from build123d import *

# Parameters (mm, degrees)
F0_R     = 8.25
F1_DEPTH = 8


with BuildPart() as f1:
    # F0 (on Top) → F1 (new body)
    with BuildSketch(Plane.XY):
        with BuildLine():
            Line((-16, 18.282857), (-16, 12))
            ThreePointArc((-16, 12), (0, -20), (16, 12))
            Line((16, 12), (16, 18.282857))
            Line((16, 18.282857), (14, 18.282857))
            Line((14, 18.282857), (14, 14.282857))
            ThreePointArc((14, 14.282857), (10.5, 13.156254), (7, 14.282857))
            Line((7, 14.282857), (7, 18.282857))
            Line((7, 18.282857), (5, 18.282857))
            Line((5, 18.282857), (5, 14.282857))
            Line((5, 14.282857), (0, 14.282857))
            Line((0, 14.282857), (-5, 14.282857))
            Line((-5, 14.282857), (-5, 18.282857))
            Line((-5, 18.282857), (-7, 18.282857))
            Line((-7, 18.282857), (-7, 14.282857))
            ThreePointArc((-7, 14.282857), (-10.5, 13.156254), (-14, 14.282857))
            Line((-14, 14.282857), (-14, 18.282857))
            Line((-14, 18.282857), (-16, 18.282857))
        make_face()
        Circle(F0_R, mode=Mode.SUBTRACT)
    extrude(amount=F1_DEPTH)


solid = f1.part
Geometry: final body of the model. Coordinates: model frame, mm. A direction names the side the tool comes from. Round coordinates to 2 decimals unless told otherwise and drop trailing zeros. Order: outer loops, then holes, each group sorted by start corner. A loop starts at its lowest first (then second) coordinate and runs counter-clockwise, first axis right, second up.
Q1. Section D-D, the plane y = 0. Output: boundary loops of the cut face in (x, z), and give its area (3 significant figures).
Result sheet:
outline: (-20, 0) - (-8.25, 0) - (-8.25, 8) - (-20, 8) - close; (8.25, 0) - (20, 0) - (20, 8) - (8.25, 8) - close
area: 188 mm2
Q2. Pin query (flat end, axial travel): pin 1 (4 mm diameter, centred on x = 2.5, z = 2.5, fed in from +Y); pin 2 (4 mm diameter, centred on x = 5, z = 3, fed in from -Y); pin 3 (1.2 mm diameter, centred on y = 16, z = 2, fed in from +X); pin 4 (13 mm diameter, centred on x = 0, y = 0, fed in from -Z). Return the tip coordinate at first contact, or that it passes through.
Result sheet:
pin 1: stops at y = 14.28
pin 2: stops at y = -19.77
pin 3: stops at x = 16
pin 4: passes through
Q3. Section A-A, the plane x = 0. Output: boundary loops of the cut face in (y, z), and give its area (3 significant figures).
Result sheet:
outline: (-20, 0) - (-8.25, 0) - (-8.25, 8) - (-20, 8) - close; (8.25, 0) - (14.28, 0) - (14.28, 8) - (8.25, 8) - close
area: 142 mm2
Q4. Section C-C, the plane z = 4. Output: boundary loops of the cut face in (x, y).
Result sheet:
outline: (-16, 12) arc R20 ccw (long way) to (16, 12) - (16, 18.28) - (14, 18.28) - (14, 14.28) arc R6 cw to (7, 14.28) - (7, 18.28) - (5, 18.28) - (5, 14.28) - (-5, 14.28) - (-5, 18.28) - (-7, 18.28) - (-7, 14.28) arc R6 cw to (-14, 14.28) - (-14, 18.28) - (-16, 18.28) - close; hole circle Ø16.5 at (0, 0)
Q5. Section B-B, the plane y = 15. Output: boundary loops of the cut face in (x, z).
Result sheet:
outline: (-16, 0) - (-14, 0) - (-14, 8) - (-16, 8) - close; (-7, 0) - (-5, 0) - (-5, 8) - (-7, 8) - close; (5, 0) - (7, 0) - (7, 8) - (5, 8) - close; (14, 0) - (16, 0) - (16, 8) - (14, 8) - close
Q6. Material intervals for probe 1 along Y at (x, z) = (0, 2); probe 2 along X at (y, z) = (1.5, 7.75); probe 3 along Y at (x, z) = (13, 2.5), sorted ascending.
Result sheet:
probe 1: y = -20 to -8.25, 8.25 to 14.28
probe 2: x = -19.94 to -8.11, 8.11 to 19.94
probe 3: y = -15.2 to 13.7
Q7. Mould query, pull axis Y, two halves, no side actions, for faces 1 (the face through (14, 16, 4)), 2 (the face through (7.62, -3.16, 3.94)), 3 (the face through (-10.448, 13.156, 3.944)), 4 (the face through (-0.62, -19.99, 3.94)). Classes: released by +Y, released by -Y, zero draft, split by the parting line, or undercut.
Result sheet:
face 1: zero draft
face 2: undercut
face 3: released by +Y
face 4: split by the parting line
Q8. Access query for faces 5 (the face through (-16, 15, 4)), 6 (the face through (-14, 16, 4)), 7 (the face through (16, 15, 4)). Directions: +Z, -Z, +X, -X, +Y, -Y. A direction counts if a zero-diameter tool reaches every point of the face in a straight line with its end or side. Return the directions, or none.
Result sheet:
face 5: +Z, -Z, -X, +Y
face 6: +Z, -Z, +Y
face 7: +Z, -Z, +X, +Y
